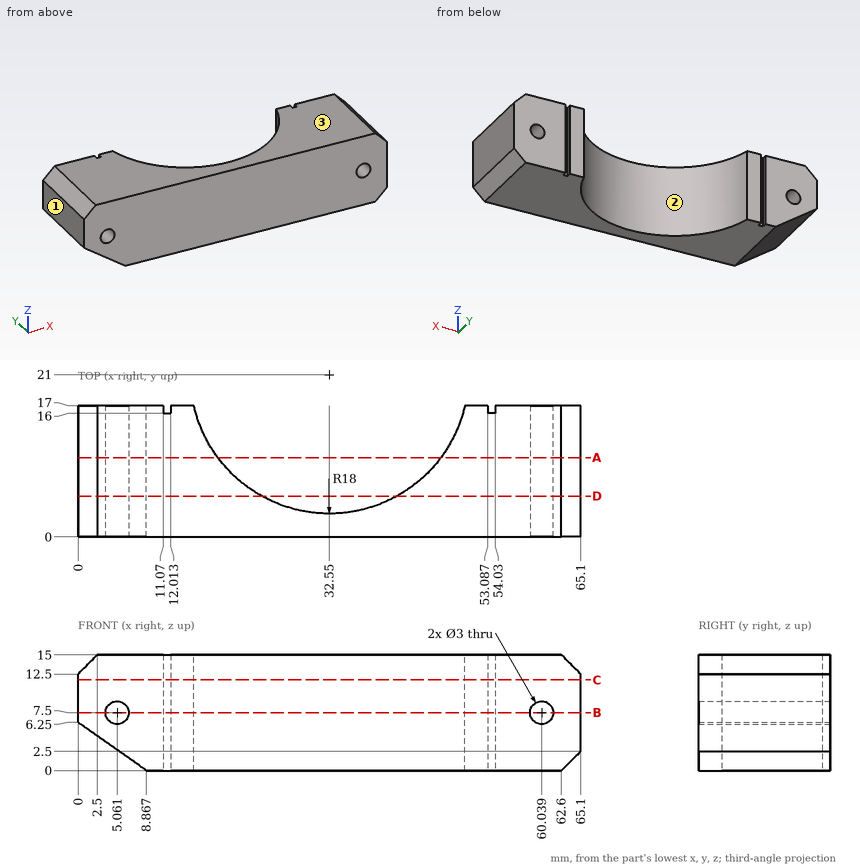
Here's the drawing with two shaded views (mm, measured from the low corner). I have some questions. Give positions to 0.01 mm unless a question says otherwise; leave off trailing zeros. Loops run counter-clockwise (first coordinate to the right, second up) from the corner with the lowest first, then second, coordinate; pieces in that order, holes last. Notation, with made-up numbers: (86.5, -9.5) -> (120.5, -9.5) arc R22 cw to (120.5, 0.5) -> close; hole circle Ø2 at (64.5, 2.25). An arc over 180 degrees is marked (long way). Answer as a JSON object with one key per item and string values. Group by question number.
Item 1: Imagine slicing it at D-D on y = 5.25. Give the number of separate pieces and of enclosed holes in the cut face, then the cut area to 3 significant figures.
Item 2: Imagine slicing it at B-B on z = 7.5. Write out the boundary of the cut face in (x, y).
Item 3: Imagine slicing it at A-A on y = 10.25. Write out the boundary of the cut face in (x, z).
Item 4: Imagine slicing it at C-C on z = 11.75. Write out the boundary of the cut face in (x, y), then the cut area to 3 significant figures.
Item 5: Will these pins go through, and if not, where does the flat tip stop? pin 1 (5 mm diameter, centred on y = 4, z = 2.5, fed in from -X) (1 decimal); pin 2 (3 mm diameter, centred on x = 47.5, z = 12, fed in from +Y) (1 decimal); pin 3 (1.5 mm diameter, centred on x = 23, y = 6.5, fed in from -Z); pin 4 (2 mm diameter, centred on x = 43, z = 13, fed in from +Y).
Item 6: I need wall thicknesses on L1, parallel to X at y = 4.5, z = 6.5 (1 decimal); L2, parallel to X at y = 14, z = 1.5 (1 decimal); L3, parallel to Y at x = 37, z = 6.25. Which ranges of each line are inside material? Lowest first, please.
Item 7: Thinking about a two-plate mould opening in X: for the marked faces 1, 2 and 3, which applies, pulls with the +X half, pulls with the -X half, needs draft (parallel to the pull), parting line crosses it, or undercut?
Answer list:
{
 "1": {"separate pieces": "2", "enclosed holes": "2", "area": "664 mm2"},
 "2": {"outline": "(0, 0) -> (3.56, 0) -> (3.56, 17) -> (0, 17) -> close; (6.56, 0) -> (58.54, 0) -> (58.54, 17) -> (54.03, 17) -> (54.03, 16) -> (53.09, 16) -> (53.09, 17) -> (50.1, 17) arc R18 cw to (15, 17) -> (12.01, 17) -> (12.01, 16) -> (11.07, 16) -> (11.07, 17) -> (6.56, 17) -> close; (61.54, 0) -> (65.1, 0) -> (65.1, 17) -> (61.54, 17) -> close"},
 "3": {"outline": "(0, 6.25) -> (8.87, 0) -> (18.11, 0) -> (18.11, 15) -> (2.5, 15) -> (0, 12.5) -> close; (46.99, 0) -> (62.6, 0) -> (65.1, 2.5) -> (65.1, 12.5) -> (62.6, 15) -> (46.99, 15) -> close; hole circle Ø3 at (5.06, 7.5); hole circle Ø3 at (60.04, 7.5)"},
 "4": {"outline": "(0, 0) -> (65.1, 0) -> (65.1, 17) -> (54.03, 17) -> (54.03, 16) -> (53.09, 16) -> (53.09, 17) -> (50.1, 17) arc R18 cw to (15, 17) -> (12.01, 17) -> (12.01, 16) -> (11.07, 16) -> (11.07, 17) -> (0, 17) -> close", "area": "739 mm2"},
 "5": {"pin 1": "stops at x = 1.8", "pin 2": "stops at y = 13.7", "pin 3": "stops at z = 0", "pin 4": "stops at y = 7.11"},
 "6": {"L1": "x = 0 to 3.9, 6.2 to 25.4, 39.7 to 58.9, 61.2 to 65.1", "L2": "x = 6.7 to 16, 49.1 to 64.1", "L3": "y = 0 to 3.56"},
 "7": {"face 1": "pulls with the -X half", "face 2": "undercut", "face 3": "needs draft"}
}
